The figure shows three views and two pictorial views of one solid part (mm, origin at its lowest corner). Answer the questions. A direction names the side the tool comes from. Give positions to 0.01 mm unless a question says otherwise; leave off trailing zeros. Order: outer loops, then holes, each group sorted by start corner. A loop starts at its lowest first (then second) coordinate and runs counter-clockwise, first axis right, second up. Notation, with made-up numbers: (-1.5, -5) - (15.5, -5) arc R17 cw to (15.5, 15) - close; hole circle Ø1 at (14.5, 33). An arc over 180 degrees is marked (long way). Answer as a JSON object with one key per item and string values. Group by question number.
Q1. Consider line 1 (X direction, y = 3.6, z = 11.75); line 2 (Z direction, x = 18.5, y = 1.2). Determine where each line is inside the solid, lowest interval first.
Q2. A cutting plane is placed at B-B, the plane y = 1.3. Give the vertices of the cut face in (x, z), and give its area (3 significant figures).
Q3. The mould has two halves that part along X. Classify the marked faces 3, 4 and 5: released by +X, released by -X, zero draft, split by the parting line, or undercut.
Q4. For the marked faces 1 and 2, determine the directions among +Z, -Z, +X, -X, +Y, -Y from which every point of the face is accessible in a straight line to the end or side of a thin tool.
Q5. Given pin 1 (3 mm diameter, centred on x = 57, y = 3.5, fed in from +Z), flat-ended and moving along its own axis, determine where the tip first touches the part or whether it passes through.
Q6. A cutting plane is placed at C-C, the plane x = 53. Give the vertices of the cut face in (y, z), and give its area (3 significant figures).
Q7. A cutting plane is placed at A-A, the plane z = 18. Give the vertices of the cut face in (x, y).
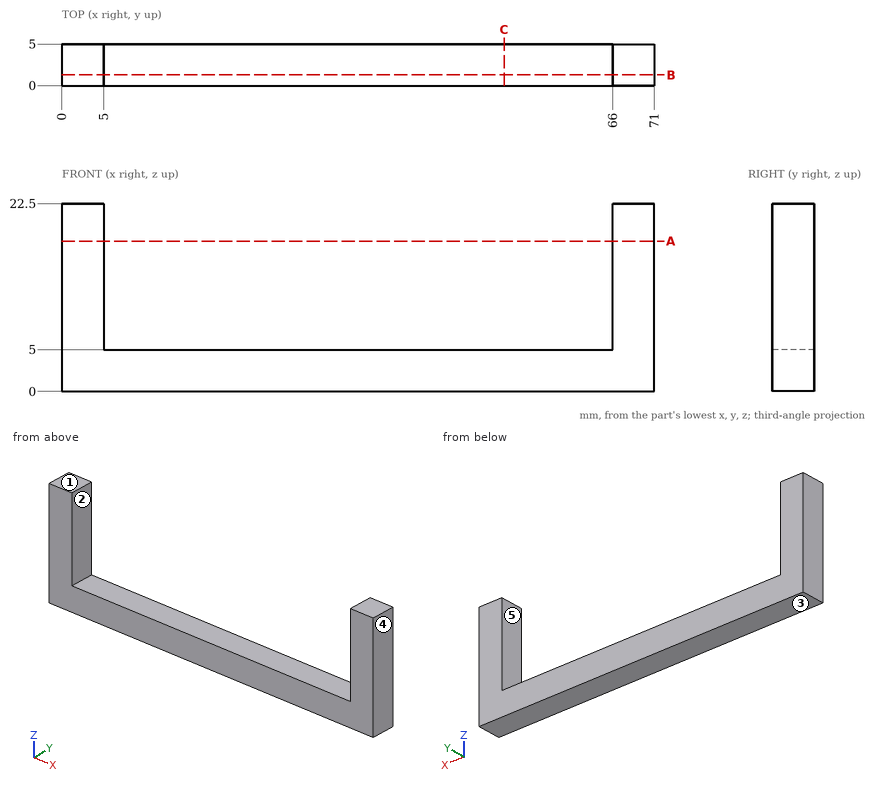
Reply:
{
 "1": {"line 1": "x = 0 to 5, 66 to 71", "line 2": "z = 0 to 5"},
 "2": {"outline": "(0, 0) - (71, 0) - (71, 22.5) - (66, 22.5) - (66, 5) - (5, 5) - (5, 22.5) - (0, 22.5) - close", "area": "530 mm^2"},
 "3": {"face 3": "zero draft", "face 4": "released by +X", "face 5": "undercut"},
 "4": {"face 1": "+Z, +X, -X, +Y, -Y", "face 2": "+Z, +Y, -Y"},
 "5": {"pin 1": "stops at z = 5"},
 "6": {"outline": "(0, 0) - (5, 0) - (5, 5) - (0, 5) - close", "area": "25.0 mm^2"},
 "7": {"outline": "(0, 0) - (5, 0) - (5, 5) - (0, 5) - close; (66, 0) - (71, 0) - (71, 5) - (66, 5) - close"}
}
